Design review of the part built by this model. Coordinates are the model's own, in mm. A direction names the side the tool comes from. Coordinates: 2 decimals unless noted, no trailing zeros. Order: outer loops, then holes, each group sorted by start corner. A loop starts at its lowest first (then second) coordinate and runs counter-clockwise, first axis right, second up. Notation, with made-up numbers: (-8.5, 2) - (14.5, 2) arc R15 ccw to (14.5, 15) - close; hole circle Ø9 at (22.25, -12.75). An arc over 180 degrees is marked (long way). Write item = value, one per line. Start each with the question number.
```python
from build123d import *

# Parameters (mm, degrees)
EXTRUDE_1_DEPTH     = 10
SKETCH_2_R          = 1.5
CUT_EXTRUDE_1_DEPTH = 10
SKETCH_3_R          = 1.5
CUT_EXTRUDE_2_DEPTH = 10


with BuildPart() as part:
    # 草图1 → 凸台-拉伸1 (new body)
    with BuildSketch(Plane(origin=(0, 0, 0), x_dir=(1, 0, 0), z_dir=(0, 1, 0))):
        Polygon((-13, 0), (0, 0), (0, 23), (-3, 23), (-3, 3), (-13, 3), align=None)
    extrude(amount=EXTRUDE_1_DEPTH)

    # 草图2 → 切除-拉伸1 (cut)
    with BuildSketch(Plane.ZY.offset(3)):
        with Locations((-18, 5)):
            Circle(SKETCH_2_R)
        with Locations((-8, 5)):
            Circle(SKETCH_2_R)
    extrude(amount=-CUT_EXTRUDE_1_DEPTH, mode=Mode.SUBTRACT)

    # 草图3 → 切除-拉伸2 (cut)
    with BuildSketch(Plane(origin=(0, 0, -3), x_dir=(-1, 0, 0), z_dir=(0, 0, -1))):
        with Locations((8, 5)):
            Circle(SKETCH_3_R)
        with Locations((-2, 5)):
            Circle(SKETCH_3_R)
    extrude(amount=-CUT_EXTRUDE_2_DEPTH, mode=Mode.SUBTRACT)


solid = part.part
```
Item 1: For line 1 (Y direction, x = -2.25, z = -8); line 2 (Z direction, x = -8.25, y = 2.75), list the stretches that pass through material, from the lowest coordinate up.
Item 2: For P1, Ø3, axis at x = -5.5, y = 6.5, coming from the -Z side, flat-tipped, find the tip position at first contact; note if it passes through.
Item 3: For faces 4 (the flat face through (-3, 5, -13)), 5 (the cylindrical face through (-6.8, 4.1, -1.5)), list the 3-axis set-ups (+Z, -Z, +X, -X, +Y, -Y) from which the entire face can be reached by the end or side of a thin tool; tool diameter is ignored.
Item 4: Add section D-D on z = -1.25. Give the boundary of the cut face in (x, y).
Item 5: Add section C-C on y = 5.75. Give the boundary of the cut face in (x, z).
Item 6: Mouldability with a two-part tool opening along Y and no side actions: class faces 1 (the flat face through (-6.8, 3.8, -3)), 2 (the flat face through (-2.7, 10, -8.1)), 3 (the cylindrical face through (-1.52, 5.07, -19.5)) as +Y half, -Y half, draft (parallel to the pull), parting line (faces both ways), or undercut.
Item 7: Add section A-A on z = -18. Give the boundary of the cut face in (x, y), plus the area to 3 significant figures.
Item 8: Add section B-B on x = -8. Give the boundary of the cut face in (y, z), plus the area to 3 significant figures.
Worked out:
q1.line_1 = 0 to 3.5, 6.5 to 10
q1.line_2 = -3 to 0
q2.P1 = -3
q3.face_4 = -Z, -X, +Y, -Y
q3.face_5 = +Z, -Z
q4.outline = (-13, 0) - (0, 0) - (0, 10) - (-13, 10) - close; hole circle Ø3 at (-8, 5)
q5.outline = (-13, -3) - (-9.3, -3) - (-9.3, 0) - (-13, 0) - close; (-6.7, -3) - (-3, -3) - (-3, -6.7) - (0, -6.7) - (0, 0) - (-6.7, 0) - close; (-3, -23) - (0, -23) - (0, -19.3) - (-3, -19.3) - close; (-3, -16.7) - (0, -16.7) - (0, -9.3) - (-3, -9.3) - close
q6.face_1 = draft
q6.face_2 = +Y half
q6.face_3 = undercut
q7.outline = (-3, 0) - (0, 0) - (0, 3.5) - (-3, 3.5) - close; (-3, 6.5) - (0, 6.5) - (0, 10) - (-3, 10) - close
q7.area = 21.0 mm2
q8.outline = (0, -3) - (3.5, -3) - (3.5, 0) - (0, 0) - close; (6.5, -3) - (10, -3) - (10, 0) - (6.5, 0) - close
q8.area = 21.0 mm2
